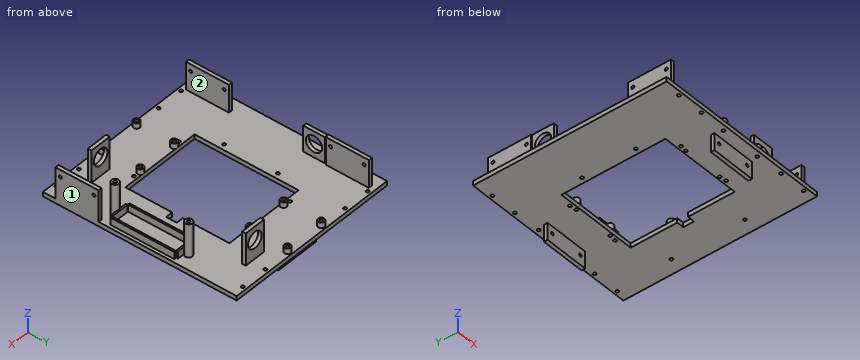
from build123d import *

# Parameters (mm, degrees)
UPPER_DECK_CENTRAL_OPENING_92X116_START       = 52
SKETCH_1_W                                    = 220
SKETCH_1_H                                    = 216
SKETCH_1_W_2                                  = 92
SKETCH_1_H_2                                  = 116
UPPER_DECK_CENTRAL_OPENING_92X116_DEPTH       = 5
EIGHT_MATCHING_M3_CLEARANCE_START             = 58
SKETCH_2_R                                    = 1.7
EIGHT_MATCHING_M3_CLEARANCE_DEPTH             = 7
CAMERA_BASE_TWO_M3_START                      = 58
SKETCH_4_R                                    = 1.7
CAMERA_BASE_TWO_M3_DEPTH                      = 7
UPPER_DECK_REAR_BOX_AND_PIVOT_CLEARANCE_START = 58
SKETCH_5_W                                    = 16
SKETCH_5_H                                    = 220
SKETCH_5_W_2                                  = 8
UPPER_DECK_REAR_BOX_AND_PIVOT_CLEARANCE_DEPTH = 7
BATTERY_CLAMP_VERTICAL_TOOL_ACCESS_DEPTH      = 70
BATTERY_CLAMP_VERTICAL_TOOL_ACCESS_DEPTH_BACK = 70
SKETCH_6_W                                    = 11
SKETCH_6_H                                    = 12
INTEGRAL_DRIVER_STANDOFFS_6MM_START           = 57
SKETCH_7_R                                    = 3.5
INTEGRAL_DRIVER_STANDOFFS_6MM_DEPTH           = 6
ELECTRONICS_MATCHING_DECK_HOLES_START         = 64
SKETCH_8_R                                    = 1.7
ELECTRONICS_MATCHING_DECK_HOLES_DEPTH         = 13
CONTROL_BATTERY_LOW_LOCATORS_START            = 57
SKETCH_9_W                                    = 2
SKETCH_9_H                                    = 71
SKETCH_9_W_2                                  = 20
SKETCH_9_H_2                                  = 2
CONTROL_BATTERY_LOW_LOCATORS_DEPTH            = 8
CONTROL_BATTERY_INTEGRAL_CLAMP_POSTS_START    = 57
SKETCH_10_R                                   = 4
CONTROL_BATTERY_INTEGRAL_CLAMP_POSTS_DEPTH    = 37
CONTROL_BATTERY_M3_THROUGH_START              = 95
SKETCH_11_R                                   = 1.7
CONTROL_BATTERY_M3_THROUGH_DEPTH              = 44
SIDE_IR_DIRECT_UNDERDECK_MOUNTS_START         = 33
SKETCH_12_W                                   = 50
SKETCH_12_H                                   = 4
SIDE_IR_DIRECT_UNDERDECK_MOUNTS_DEPTH         = 19
SIDE_IR_37P4_PITCH_DEPTH                      = 110
SIDE_IR_37P4_PITCH_DEPTH_BACK                 = 110
SKETCH_13_R                                   = 1.7
FRONT_IR_DIRECT_UPPER_MOUNTS_START            = 57
SKETCH_14_W                                   = 4
SKETCH_14_H                                   = 48
FRONT_IR_DIRECT_UPPER_MOUNTS_DEPTH            = 31
FRONT_IR_M3_MOUNTS_START                      = -87
SKETCH_15_R                                   = 1.7
FRONT_IR_M3_MOUNTS_DEPTH                      = 4
REAR_IR_ABOVE_TAIL_NOT_ON_RAMP_START          = 57
SKETCH_16_W                                   = 4
SKETCH_16_H                                   = 48
REAR_IR_ABOVE_TAIL_NOT_ON_RAMP_DEPTH          = 35
REAR_IR_M3_MOUNTS_START                       = 96
SKETCH_17_R                                   = 1.7
REAR_IR_M3_MOUNTS_DEPTH                       = 4
FRONT_PHOTOEYE_SHORT_DIRECT_SEAT_START        = 57
SKETCH_18_W                                   = 4
SKETCH_18_H                                   = 24
FRONT_PHOTOEYE_SHORT_DIRECT_SEAT_DEPTH        = 29
FRONT_M18_CLEARANCE_START                     = -88
SKETCH_19_R                                   = 9.1
FRONT_M18_CLEARANCE_DEPTH                     = 4
SIDE_PHOTOEYE_DIRECT_SEATS_START              = 57
SKETCH_20_W                                   = 24
SKETCH_20_H                                   = 4
SIDE_PHOTOEYE_DIRECT_SEATS_DEPTH              = 36
SIDE_M18_CLEARANCES_DEPTH                     = 110
SIDE_M18_CLEARANCES_DEPTH_BACK                = 110
SKETCH_21_R                                   = 9.1


with BuildPart() as part:
    # 草图1 → Upper_deck_central_opening_92x116 (new body)
    with BuildSketch(Plane.XY.offset(UPPER_DECK_CENTRAL_OPENING_92X116_START)):
        Rectangle(SKETCH_1_W, SKETCH_1_H)
        Rectangle(SKETCH_1_W_2, SKETCH_1_H_2, mode=Mode.SUBTRACT)
    extrude(amount=UPPER_DECK_CENTRAL_OPENING_92X116_DEPTH)

    # 草图2 → Eight_matching_M3_clearance (cut)
    with BuildSketch(Plane.XY.offset(EIGHT_MATCHING_M3_CLEARANCE_START)):
        with Locations(Location((-83, -104, 0), (0, 0, 180))):
            Circle(SKETCH_2_R)
        with Locations(Location((-83, 104, 0), (0, 0, 180))):
            Circle(SKETCH_2_R)
        with Locations(Location((-53, -104, 0), (0, 0, 180))):
            Circle(SKETCH_2_R)
        with Locations(Location((-53, 104, 0), (0, 0, 180))):
            Circle(SKETCH_2_R)
        with Locations(Location((53, -104, 0), (0, 0, 180))):
            Circle(SKETCH_2_R)
        with Locations(Location((53, 104, 0), (0, 0, 180))):
            Circle(SKETCH_2_R)
        with Locations(Location((83, -104, 0), (0, 0, 180))):
            Circle(SKETCH_2_R)
        with Locations(Location((83, 104, 0), (0, 0, 180))):
            Circle(SKETCH_2_R)
    extrude(amount=-EIGHT_MATCHING_M3_CLEARANCE_DEPTH, mode=Mode.SUBTRACT)

    # 草图4 → Camera_base_two_M3 (cut)
    with BuildSketch(Plane.XY.offset(CAMERA_BASE_TWO_M3_START)):
        with Locations(Location((-52, -30, 0), (0, 0, 180))):
            Circle(SKETCH_4_R)
        with Locations(Location((-52, 30, 0), (0, 0, 180))):
            Circle(SKETCH_4_R)
    extrude(amount=-CAMERA_BASE_TWO_M3_DEPTH, mode=Mode.SUBTRACT)

    # 草图5 → Upper_deck_rear_box_and_pivot_clearance (cut)
    with BuildSketch(Plane.XY.offset(UPPER_DECK_REAR_BOX_AND_PIVOT_CLEARANCE_START)):
        with Locations((104, 0)):
            Rectangle(SKETCH_5_W, SKETCH_5_H)
        with Locations((-108, 0)):
            Rectangle(SKETCH_5_W_2, SKETCH_5_H)
    extrude(amount=-UPPER_DECK_REAR_BOX_AND_PIVOT_CLEARANCE_DEPTH, mode=Mode.SUBTRACT)

    # 草图6 → Battery_clamp_vertical_tool_access (cut, two sides: drawn at the far end of the back side and taken through both)
    with BuildSketch(Plane.XY.offset(-BATTERY_CLAMP_VERTICAL_TOOL_ACCESS_DEPTH_BACK)):
        with Locations((48.5, 0)):
            Rectangle(SKETCH_6_W, SKETCH_6_H)
    extrude(amount=BATTERY_CLAMP_VERTICAL_TOOL_ACCESS_DEPTH + BATTERY_CLAMP_VERTICAL_TOOL_ACCESS_DEPTH_BACK, mode=Mode.SUBTRACT)

    # 草图7 → Integral_driver_standoffs_6mm (add)
    with BuildSketch(Plane.XY.offset(INTEGRAL_DRIVER_STANDOFFS_6MM_START)):
        with Locations(Location((-22.5, -103, 0), (0, 0, 180))):
            Circle(SKETCH_7_R)
        with Locations(Location((-22.5, -61, 0), (0, 0, 121.002719134))):
            Circle(SKETCH_7_R)
        with Locations(Location((22.5, -103, 0), (0, 0, 180))):
            Circle(SKETCH_7_R)
        with Locations(Location((22.5, -61, 0), (0, 0, 121.002719134))):
            Circle(SKETCH_7_R)
        with Locations(Location((-22.5, 61, 0), (0, 0, 238.997280866))):
            Circle(SKETCH_7_R)
        with Locations(Location((-22.5, 103, 0), (0, 0, 180))):
            Circle(SKETCH_7_R)
        with Locations(Location((22.5, 61, 0), (0, 0, 238.997280866))):
            Circle(SKETCH_7_R)
        with Locations(Location((22.5, 103, 0), (0, 0, 180))):
            Circle(SKETCH_7_R)
    extrude(amount=INTEGRAL_DRIVER_STANDOFFS_6MM_DEPTH)

    # 草图8 → Electronics_matching_deck_holes (cut)
    with BuildSketch(Plane.XY.offset(ELECTRONICS_MATCHING_DECK_HOLES_START)):
        with Locations((-22.5, -103)):
            Circle(SKETCH_8_R)
        with Locations((-22.5, -61)):
            Circle(SKETCH_8_R)
        with Locations((22.5, -103)):
            Circle(SKETCH_8_R)
        with Locations((22.5, -61)):
            Circle(SKETCH_8_R)
        with Locations((-22.5, 61)):
            Circle(SKETCH_8_R)
        with Locations((-22.5, 103)):
            Circle(SKETCH_8_R)
        with Locations((22.5, 61)):
            Circle(SKETCH_8_R)
        with Locations((22.5, 103)):
            Circle(SKETCH_8_R)
        with Locations((-30, -62)):
            Circle(SKETCH_8_R)
        with Locations((-30, 62)):
            Circle(SKETCH_8_R)
        with Locations((30, -62)):
            Circle(SKETCH_8_R)
        with Locations((30, 62)):
            Circle(SKETCH_8_R)
    extrude(amount=-ELECTRONICS_MATCHING_DECK_HOLES_DEPTH, mode=Mode.SUBTRACT)

    # 草图9 → Control_battery_low_locators (add)
    with BuildSketch(Plane.XY.offset(CONTROL_BATTERY_LOW_LOCATORS_START)):
        with Locations((68.5, 0)):
            Rectangle(SKETCH_9_W, SKETCH_9_H)
        with Locations((91.5, 0)):
            Rectangle(SKETCH_9_W, SKETCH_9_H)
        with Locations((80, -36.5)):
            Rectangle(SKETCH_9_W_2, SKETCH_9_H_2)
        with Locations((80, 36.5)):
            Rectangle(SKETCH_9_W_2, SKETCH_9_H_2)
    extrude(amount=CONTROL_BATTERY_LOW_LOCATORS_DEPTH)

    # 草图10 → Control_battery_integral_clamp_posts (add)
    with BuildSketch(Plane.XY.offset(CONTROL_BATTERY_INTEGRAL_CLAMP_POSTS_START)):
        with Locations(Location((80, -41, 0), (0, 0, 118.955024372))):
            Circle(SKETCH_10_R)
        with Locations(Location((80, 41, 0), (0, 0, 241.044975628))):
            Circle(SKETCH_10_R)
    extrude(amount=CONTROL_BATTERY_INTEGRAL_CLAMP_POSTS_DEPTH)

    # 草图11 → Control_battery_M3_through (cut)
    with BuildSketch(Plane.XY.offset(CONTROL_BATTERY_M3_THROUGH_START)):
        with Locations((80, -41)):
            Circle(SKETCH_11_R)
        with Locations((80, 41)):
            Circle(SKETCH_11_R)
    extrude(amount=-CONTROL_BATTERY_M3_THROUGH_DEPTH, mode=Mode.SUBTRACT)

    # 草图12 → Side_IR_direct_underdeck_mounts (add)
    with BuildSketch(Plane.XY.offset(SIDE_IR_DIRECT_UNDERDECK_MOUNTS_START)):
        with Locations((0, 93)):
            Rectangle(SKETCH_12_W, SKETCH_12_H)
        with Locations((0, -93)):
            Rectangle(SKETCH_12_W, SKETCH_12_H)
    extrude(amount=SIDE_IR_DIRECT_UNDERDECK_MOUNTS_DEPTH)

    # 草图13 → Side_IR_37p4_pitch (cut, two sides: drawn at the far end of the back side and taken through both)
    with BuildSketch(Plane(origin=(0, 0, 0), x_dir=(1, 0, 0), z_dir=(0, 1, 0)).offset(-SIDE_IR_37P4_PITCH_DEPTH_BACK)):
        with Locations(Location((-18.7, -44, 0), (0, 0, 90))):
            Circle(SKETCH_13_R)
        with Locations(Location((18.7, -44, 0), (0, 0, 90))):
            Circle(SKETCH_13_R)
    extrude(amount=SIDE_IR_37P4_PITCH_DEPTH + SIDE_IR_37P4_PITCH_DEPTH_BACK, mode=Mode.SUBTRACT)

    # 草图14 → Front_IR_direct_upper_mounts (add)
    with BuildSketch(Plane.XY.offset(FRONT_IR_DIRECT_UPPER_MOUNTS_START)):
        with Locations((-89, -78)):
            Rectangle(SKETCH_14_W, SKETCH_14_H)
        with Locations((-89, 78)):
            Rectangle(SKETCH_14_W, SKETCH_14_H)
    extrude(amount=FRONT_IR_DIRECT_UPPER_MOUNTS_DEPTH)

    # 草图15 → Front_IR_M3_mounts (cut)
    with BuildSketch(Plane(origin=(0, 0, 0), x_dir=(0, 0, -1), z_dir=(1, 0, 0)).offset(FRONT_IR_M3_MOUNTS_START)):
        with Locations((-80, -96.7)):
            Circle(SKETCH_15_R)
        with Locations((-80, -59.3)):
            Circle(SKETCH_15_R)
        with Locations((-80, 59.3)):
            Circle(SKETCH_15_R)
        with Locations((-80, 96.7)):
            Circle(SKETCH_15_R)
    extrude(amount=-FRONT_IR_M3_MOUNTS_DEPTH, mode=Mode.SUBTRACT)

    # 草图16 → Rear_IR_above_tail_not_on_ramp (add)
    with BuildSketch(Plane.XY.offset(REAR_IR_ABOVE_TAIL_NOT_ON_RAMP_START)):
        with Locations((94, -70)):
            Rectangle(SKETCH_16_W, SKETCH_16_H)
    extrude(amount=REAR_IR_ABOVE_TAIL_NOT_ON_RAMP_DEPTH)

    # 草图17 → Rear_IR_M3_mounts (cut)
    with BuildSketch(Plane(origin=(0, 0, 0), x_dir=(0, 0, -1), z_dir=(1, 0, 0)).offset(REAR_IR_M3_MOUNTS_START)):
        with Locations((-84, -88.7)):
            Circle(SKETCH_17_R)
        with Locations((-84, -51.3)):
            Circle(SKETCH_17_R)
    extrude(amount=-REAR_IR_M3_MOUNTS_DEPTH, mode=Mode.SUBTRACT)

    # 草图18 → Front_photoeye_short_direct_seat (add)
    with BuildSketch(Plane.XY.offset(FRONT_PHOTOEYE_SHORT_DIRECT_SEAT_START)):
        with Locations((-90, 40)):
            Rectangle(SKETCH_18_W, SKETCH_18_H)
    extrude(amount=FRONT_PHOTOEYE_SHORT_DIRECT_SEAT_DEPTH)

    # 草图19 → Front_M18_clearance (cut)
    with BuildSketch(Plane(origin=(0, 0, 0), x_dir=(0, 0, -1), z_dir=(1, 0, 0)).offset(FRONT_M18_CLEARANCE_START)):
        with Locations((-72, 40)):
            Circle(SKETCH_19_R)
    extrude(amount=-FRONT_M18_CLEARANCE_DEPTH, mode=Mode.SUBTRACT)

    # 草图20 → Side_photoeye_direct_seats (add)
    with BuildSketch(Plane.XY.offset(SIDE_PHOTOEYE_DIRECT_SEATS_START)):
        with Locations((48, 86)):
            Rectangle(SKETCH_20_W, SKETCH_20_H)
        with Locations((48, -86)):
            Rectangle(SKETCH_20_W, SKETCH_20_H)
    extrude(amount=SIDE_PHOTOEYE_DIRECT_SEATS_DEPTH)

    # 草图21 → Side_M18_clearances (cut, two sides: drawn at the far end of the back side and taken through both)
    with BuildSketch(Plane(origin=(0, 0, 0), x_dir=(1, 0, 0), z_dir=(0, 1, 0)).offset(-SIDE_M18_CLEARANCES_DEPTH_BACK)):
        with Locations(Location((48, -78, 0), (0, 0, 90))):
            Circle(SKETCH_21_R)
    extrude(amount=SIDE_M18_CLEARANCES_DEPTH + SIDE_M18_CLEARANCES_DEPTH_BACK, mode=Mode.SUBTRACT)


solid = part.part
Verification items for the finished model (mm, model axes). Face numbers are marked on the shaded views. A direction names the side the tool comes from. Coordinates: 2 decimals unless noted, no trailing zeros. Write each loop counter-clockwise with the first axis right and the second up, starting at its lowest first coordinate (ties: lowest second). Pieces come first, ordered by that corner, then holes. Notation, with made-up numbers: (89.25, 65) - (108.25, 65) arc R13 ccw to (108.25, 69) - close; hole circle Ø8 at (37.5, 61). An arc over 180 degrees is marked (long way). Answer as a JSON object with one key per item and string values.
(1) Cross-section at A-A on y = 79. Record the cut outline in (x, z).
Report:
{"outline": "(-104, 52) - (96, 52) - (96, 57) - (-87, 57) - (-87, 88) - (-91, 88) - (-91, 57) - (-104, 57) - close"}
(2) Cross-section at D-D on x = -67. Record the cut outline in (y, z), plus the area to 3 significant figures.
Report:
{"outline": "(-108, 52) - (108, 52) - (108, 57) - (-108, 57) - close", "area": "1,080 mm^2"}
(3) Tool access check on the marked faces 1 and 2. Record the directions out of +Z, -Z, +X, -X, +Y, -Y that give a thin tool (end or side, any length) a straight path to the whole face; none if there is none.
Report:
{"face 1": "+Z, -Z, +X, +Y, -Y", "face 2": "+Z, +Y, -Y"}
(4) Cross-section at B-B on y = -10. Record the cut outline in (x, z).
Report:
{"outline": "(-104, 52) - (-46, 52) - (-46, 57) - (-104, 57) - close; (46, 52) - (96, 52) - (96, 57) - (92.5, 57) - (92.5, 65) - (90.5, 65) - (90.5, 57) - (69.5, 57) - (69.5, 65) - (67.5, 65) - (67.5, 57) - (46, 57) - close"}
(5) Thickness scan on line 1 along Y through (x, z) = (-90.35, 72); line 2 along X through (y, z) = (-83, 60); line 3 along Y through (x, z) = (0.5, 53). Record the ranges inside material, lowest first.
Report:
{"line 1": "-102 to -54, 28 to 30.9, 49.1 to 52, 54 to 102", "line 2": "-91 to -87, 92 to 96", "line 3": "-108 to -58, 58 to 108"}
(6) Cross-section at C-C on z = 71.5. Give the number of separate pieces and of enclosed holes in the cut face, plus the area to 3 significant figures.
Report:
{"separate pieces": "11", "enclosed holes": "2", "area": "772 mm^2"}
(7) Gauge pin test, flat ends, axial feed: pin 1 Ø5.5 at (x, z) = (18.7, 44) entering from -Y; pin 2 Ø5.5 at (x, y) = (-22.5, -103) entering from -Z; pin 3 Ø19 at (x, z) = (50, 74) entering from -Y. Record the tip position at first contact, or that the pin passes through.
Report:
{"pin 1": "y = -95", "pin 2": "z = 52", "pin 3": "y = -88"}
